Geometry: see drawing. Coordinates: mm, zero at the bounding-box minimum. A direction names the side the tool comes from. Round coordinates to 2 decimals unless told otherwise and drop trailing zeros. Write each loop counter-clockwise with the first axis right and the second up, starting at its lowest first coordinate (ties: lowest second). Pieces come first, ordered by that corner, then holes. Notation, with made-up numbers: (24.25, 89) -> (32.25, 89) arc R22 cw to (32.25, 106) -> close; hole circle Ø11 at (7.25, 54). An arc over 180 degrees is marked (long way). Use CSV: the item, a comma, the result in double quotes.
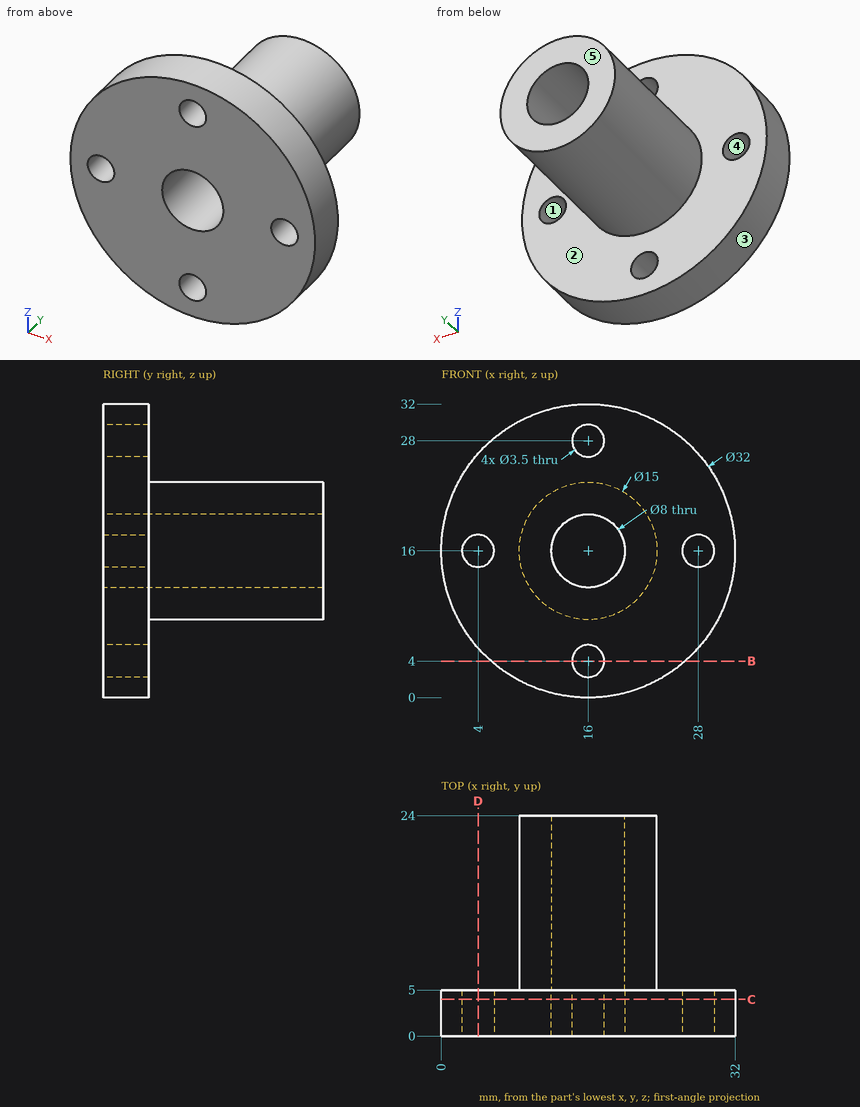
Item 1: First-contact query: pin 1 Ø5 at (x, z) = (16, 16) entering from -Y; pin 2 Ø4 at (y, z) = (3.5, 7) entering from -X; pin 3 Ø5.5 at (x, z) = (16, 28) entering from -Y; pin 4 Ø2 at (x, y) = (22.5, 20.5) entering from -Z. Flat tips, straight axial feed; report the tip coordinate or a pass-through.
Worked answers:
pin 1,"passes through"
pin 2,"stops at x = 1.61"
pin 3,"stops at y = 0"
pin 4,"stops at z = 10.9"
Item 2: Section query D-D on x = 4. Return the cut outline in (y, z).
Worked answers:
outline,"(0, 5.42) -> (5, 5.42) -> (5, 14.25) -> (0, 14.25) -> close; (0, 17.75) -> (5, 17.75) -> (5, 26.58) -> (0, 26.58) -> close"
Item 3: Line query: line 1 (Z direction, x = 16, y = 3.6); line 2 (Z direction, x = 16, y = 12). Output: solid intervals per line, ascending.
Worked answers:
line 1,"z = 0 to 2.25, 5.75 to 12, 20 to 26.25, 29.75 to 32"
line 2,"z = 8.5 to 12, 20 to 23.5"
Item 4: Set-up query: the marked faces 1 and 2. Return all of +Z, -Z, +X, -X, +Y, -Y with unobstructed straight access to the full face (end or side cutting, diameter ignored); none if empty.
Worked answers:
face 1,"+Y, -Y"
face 2,"+Y"
Item 5: Section query B-B on z = 4. Return the cut outline in (x, y), plus the area to 3 significant figures.
Worked answers:
outline,"(5.42, 0) -> (14.25, 0) -> (14.25, 5) -> (5.42, 5) -> close; (17.75, 0) -> (26.58, 0) -> (26.58, 5) -> (17.75, 5) -> close"
area,"88.3 mm²"
Item 6: Section query C-C on y = 4. Return the cut outline in (x, z), plus the area to 3 significant figures.
Worked answers:
outline,"circle Ø32 at (16, 16); hole circle Ø3.5 at (4, 16); hole circle Ø8 at (16, 16); hole circle Ø3.5 at (16, 4); hole circle Ø3.5 at (16, 28); hole circle Ø3.5 at (28, 16)"
area,"715 mm²"
Item 7: Pull-direction query (Z, two-part tool) for the marked faces 3, 4 and 5; classes: +Z half, -Z half, draft (parallel to the pull), parting line (faces both ways), or undercut.
Worked answers:
face 3,"parting line"
face 4,"undercut"
face 5,"draft"
